Autodesk Inventor part; units mm, degrees
ref_plane "YZ Plane" through (0, 0, 0) normal (1, 0, 0) x (0, 1, 0)
ref_plane "XZ Plane" through (0, 0, 0) normal (0, 1, 0) x (-1, 0, 0)
ref_plane "XY Plane" through (0, 0, 0) normal (0, 0, 1) x (1, 0, 0)
sketch "Sketch1" plane through (0, 0, 0) normal (0, 0, 1) x (1, 0, 0)
  line L0 (0, 0) -> (0, 31.75)
  line L1 (0, 31.75) -> (10.16, 31.75)
  line L2 (10.16, 31.75) -> (10.16, 7.62)
  line L3 (10.16, 7.62) -> (15.748, 7.62)
  line L4 (15.748, 7.62) -> (15.748, 18.034)
  line L5 (15.748, 18.034) -> (23.368, 18.034)
  line L6 (23.368, 18.034) -> (23.368, 7.62)
  line L7 (23.368, 7.62) -> (105.283, 7.62)
  line L8 (105.283, 7.62) -> (105.283, 18.034)
  line L9 (105.283, 18.034) -> (112.903, 18.034)
  line L10 (112.903, 18.034) -> (112.903, 7.62)
  line L11 (112.903, 7.62) -> (123.571, 7.62)
  line L12 (123.571, 7.62) -> (123.571, 31.75)
  line L13 (123.571, 31.75) -> (133.731, 31.75)
  circle A0 centre (109.093, 14.224) radius 1.778
  circle A1 centre (5.588, 25.4) radius 1.905
  line L14 (133.731, 31.75) -> (133.731, 0)
  line L15 (133.731, 0) -> (0, 0)
  circle A2 centre (128.143, 25.4) radius 1.905
  circle A3 centre (19.558, 14.224) radius 1.778
  circle A4 centre (63.5, 4.064) radius 1.905
  dimension "d0" = 31.75
  dimension "d1" = 10.16
  dimension "d2" = 24.13
  dimension "d3" = 5.588
  dimension "d19" = 10.414
  dimension "d20" = 7.62
  dimension "d21" = 10.414
  dimension "d23" = 81.915
  dimension "d24" = 10.414
  dimension "d25" = 7.62
  dimension "d26" = 10.414
  dimension "d27" = 10.668
  dimension "d28" = 24.13
  dimension "d29" = 10.16
  dimension "d30" = 3.556
  dimension "d31" = 3.81
  dimension "d33" = 133.731
  dimension "d34" = 3.81
  dimension "d37" = 3.556
  dimension "d42" = 3.81
  dimension "d57" = 63.5
  dimension "d58" = 25.4
sketch "Sketch2" plane through (0, 0, 0) normal (0, 0, 1) x (1, 0, 0)
  line L0 (15.748, 7.62) -> (10.16, 7.62)
  line L1 (12.954, 7.62) -> (117.9845, 7.62)
  line L2 (117.9845, 7.62) -> (117.9845, 21.0811)
  line L3 (117.9845, 21.0811) -> (12.954, 21.0811)
  line L4 (12.954, 21.0811) -> (12.954, 7.62)
  point P0 (0, 0)
extrude "Extrusion4" add sketch "Sketch1" along normal blind 13.081
extrude "Extrusion5" cut sketch "Sketch2" along normal blind 11.176
sketch "Sketch3" plane through (0, 0, 0) normal (1, 0, 0) x (0, 1, 0)
  line L0 (31.75, 13.081) -> (0, 13.081)
  line L1 (19.9646, 13.081) -> (19.9646, 28.448)
  line L2 (19.9646, 28.448) -> (9.7883, 28.448)
  line L3 (9.7883, 28.448) -> (9.7883, 13.081)
  circle A0 centre (14.8765, 24.9237) radius 1.778
  point P0 (0, 0)
  dimension "d47" = 15.367
  dimension "d48" = 3.556
extrude "Extrusion6" add sketch "Sketch3" along normal blind 2.032
ref_plane "Work Plane2" through (133.731, 0, 0) normal (1, 0, 0) x (0, 0, -1)
sketch "Sketch4" plane through (133.731, 0, 0) normal (1, 0, 0) x (0, 0, -1)
  line L0 (-13.081, 9.7883) -> (-28.448, 9.7883)
  line L1 (-28.448, 9.7883) -> (-28.448, 19.9646)
  line L2 (-13.081, 9.7883) -> (-28.448, 9.7883)
  line L3 (-28.448, 9.7883) -> (-28.448, 19.9646)
  line L4 (-28.448, 19.9646) -> (-13.081, 19.9646)
  line L5 (-28.448, 19.9646) -> (-13.081, 19.9646)
  line L6 (-13.081, 19.9646) -> (-13.081, 9.7883)
  line L7 (-13.081, 7.62) -> (-13.081, 18.034)
  circle A0 centre (-24.9237, 14.8765) radius 1.778
  circle A1 centre (-24.9237, 14.8765) radius 1.778
  point P0 (0, 0)
extrude "Extrusion8" add sketch "Sketch4" against normal blind 2.032
ref_plane "Work Plane3" through (0, 0, 0) normal (0, 0, -1) x (-1, 0, 0)
sketch "Sketch5" plane through (0, 0, 0) normal (0, 0, -1) x (-1, 0, 0)
  circle A0 centre (-5.588, 25.4) radius 2.413
  circle A1 centre (-63.5, 4.064) radius 1.905
  circle A2 centre (-63.5, 4.064) radius 2.286
  circle A3 centre (-128.1215, 25.4) radius 2.413
  point P0 (0, 0)
  dimension "d60" = 4.826
  dimension "d61" = 4.572
  dimension "d62" = 4.826
extrude "Extrusion9" cut sketch "Sketch5" against normal blind 15.24 contours A0 | A1 | A3
properties part number "PC_bottom_piece"
Check sheet for the modelled part. Datum: model origin and axes. Units: mm. A direction names the side the tool comes from. Coordinates: 2 decimals unless noted, no trailing zeros. Loops run counter-clockwise (first coordinate to the right, second up) from the corner with the lowest first, then second, coordinate; pieces in that order, holes last.
1) Material ranges on probe 1 along X at (y, z) = (16, 20.5); probe 2 along X at (y, z) = (8, 1.5); probe 3 along Z at (x, y) = (10, 23.5), recorded low to high.
2) Gauge pin test, flat ends, axial feed: pin 1 (12 mm diameter, centred on x = 31.5, z = 21.5, fed in from +Y); pin 2 (8 mm diameter, centred on x = 86.5, y = 6.5, fed in from +Z); pin 3 (1 mm diameter, centred on x = 1, z = 18.5, fed in from +Y); pin 4 (0.6 mm diameter, centred on x = 1, z = 19.5, fed in from -Y). Record the tip position at first contact, or that the pin passes through.
3) Sectioned sample at B-B (x = 63.5). Record the boundary of the cut face in (y, z).
4) Sectioned sample at D-D (z = 3.25). Count the separate pieces of the cut face and the enclosed holes in it, and give its area (3 significant figures).
5) Release check for a two-part mould opening along X. For faces 1 (the face through (0, 16, 11)), 2 (the face through (1, 13.1, 24.85)), 3 (the face through (10.16, 20, 6)) record: released by +X, released by -X, zero draft, split by the parting line, or undercut.
6) Access from +Z, -Z, +X, -X, +Y, -Y to the whole of each face (thin tool, end or side, straight path). Record for faces 4 (the face through (2.032, 15, 21)), 5 (the face through (109, 12, 11.176)), 6 (the face through (20.38, 15.8, 12.12)), 7 (the face through (123.571, 20, 6)).
7) Sectioned sample at A-A (z = 16.5). Record the boundary of the cut face in (x, y).
8) Sectioned sample at C-C (y = 25.4). Record the boundary of the cut face in (x, z) (1 decimal).
Check sheet entries:
1. probe 1: x = 0 to 2.03, 131.7 to 133.73
1. probe 2: x = 0 to 10.16, 123.57 to 133.73
1. probe 3: z = 0 to 13.08
2. pin 1: passes through
2. pin 2: stops at z = 13.08
2. pin 3: stops at y = 19.96
2. pin 4: stops at y = 9.79
3. outline: (0, 0) - (2.16, 0) - (2.16, 13.08) - (0, 13.08) - close; (5.97, 0) - (7.62, 0) - (7.62, 13.08) - (5.97, 13.08) - close
4. separate pieces: 1
4. enclosed holes: 3
4. area: 1,460 mm2
5. face 1: released by -X
5. face 2: zero draft
5. face 3: undercut
6. face 4: +Z, +Y, -Y
6. face 5: -Z, +Y
6. face 6: +Z, -Z
6. face 7: +Z, -Z, +Y
7. outline: (0, 9.79) - (2.03, 9.79) - (2.03, 19.96) - (0, 19.96) - close; (131.7, 9.79) - (133.73, 9.79) - (133.73, 19.96) - (131.7, 19.96) - close
8. outline: (0, 0) - (3.2, 0) - (3.2, 13.1) - (0, 13.1) - close; (8, 0) - (10.2, 0) - (10.2, 13.1) - (8, 13.1) - close; (123.6, 0) - (125.7, 0) - (125.7, 13.1) - (123.6, 13.1) - close; (130.5, 0) - (133.7, 0) - (133.7, 13.1) - (130.5, 13.1) - close
